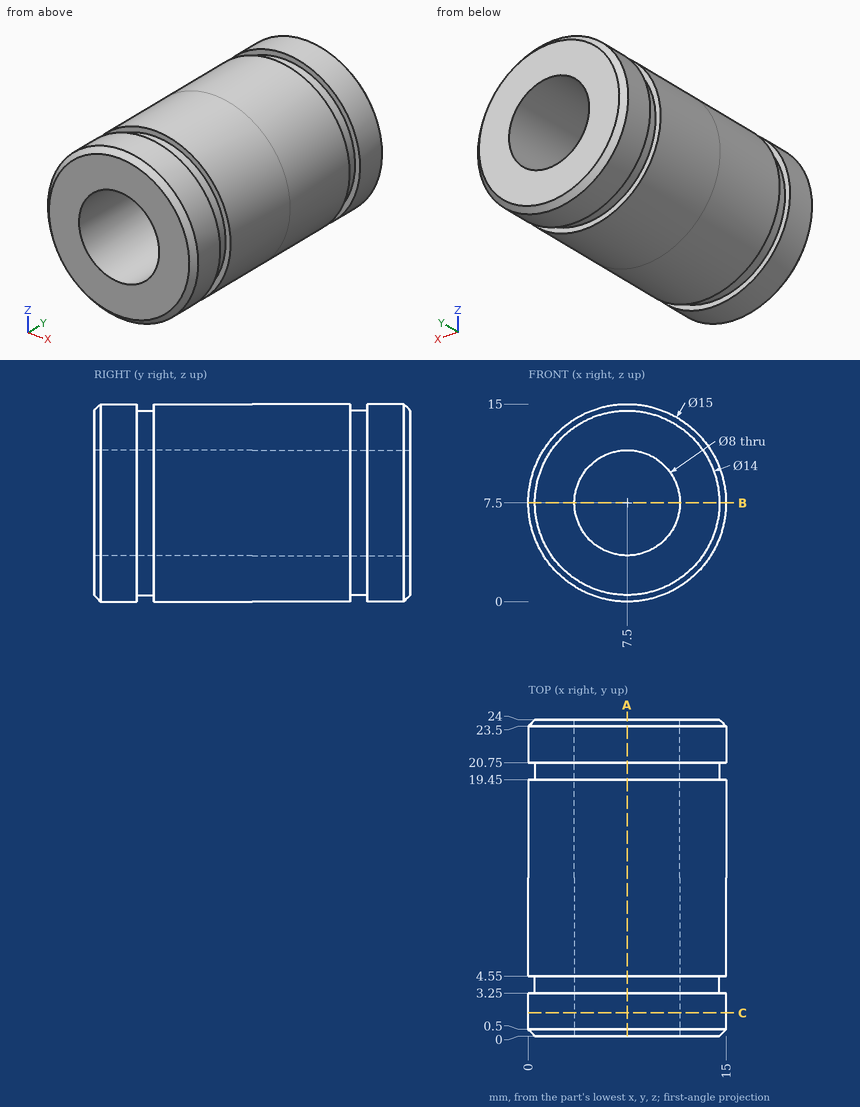
Verification items for this drawing (mm, ordinates from the low corner). Coordinates: 2 decimals unless noted, no trailing zeros. Order: outer loops, then holes, each group sorted by start corner. A loop starts at its lowest first (then second) coordinate and runs counter-clockwise, first axis right, second up. Notation, with made-up numbers: M 51,22 L 107,22 A18 ccw 107,53 Z; hole C 45.5,14 d7. An arc over 180 degrees is marked long. One line per item, written item: value. Start each with the question number.
Item 1: Sectioned sample at B-B on z = 7.5. Record the cut outline in (x, y), then the cut area to 3 significant figures.
Item 2: Sectioned sample at A-A on x = 7.5. Record the cut outline in (y, z).
Item 3: Sectioned sample at C-C on y = 1.75. Record the cut outline in (x, z), then the cut area to 3 significant figures.
Item 4: Thickness scan on probe 1 along X at (y, z) = (18.75, 7.5); probe 2 along Y at (x, z) = (2.25, 2.75); probe 3 along Y at (x, z) = (13.75, 11.25). Record the ranges inside material, lowest first.
Item 5: Depth check by flat-ended pin: P1, Ø1.5, axis at y = 15.5, z = 4.5, coming from the +X side; P2, Ø2, axis at x = 6.5, z = 9.5, coming from the -Y side; P3, Ø5, axis at x = 4, y = 6, coming from the +Z side; P4, Ø3, axis at x = 9.5, z = 5, coming from the +Y side. Enter the tip coordinate at first touch or a pass-through.
Calculated:
1. outline: M 0,0.5 L 0.5,0 L 3.5,0 L 3.5,24 L 0.5,24 L 0,23.5 L 0,20.75 L 0.5,20.75 L 0.5,19.45 L 0,19.45 L 0,4.55 L 0.5,4.55 L 0.5,3.25 L 0,3.25 Z; M 11.5,0 L 14.5,0 L 15,0.5 L 15,3.25 L 14.5,3.25 L 14.5,4.55 L 15,4.55 L 15,19.45 L 14.5,19.45 L 14.5,20.75 L 15,20.75 L 15,23.5 L 14.5,24 L 11.5,24 Z
1. area: 165 mm^2
2. outline: M 0,0.5 L 0.5,0 L 3.25,0 L 3.25,0.5 L 4.55,0.5 L 4.55,0 L 19.45,0 L 19.45,0.5 L 20.75,0.5 L 20.75,0 L 23.5,0 L 24,0.5 L 24,3.5 L 0,3.5 Z; M 0,11.5 L 24,11.5 L 24,14.5 L 23.5,15 L 20.75,15 L 20.75,14.5 L 19.45,14.5 L 19.45,15 L 4.55,15 L 4.55,14.5 L 3.25,14.5 L 3.25,15 L 0.5,15 L 0,14.5 Z
3. outline: C 7.5,7.5 d15; hole C 7.5,7.5 d8
3. area: 126 mm^2
4. probe 1: 0 to 3.5, 11.5 to 15
4. probe 2: 0.08 to 3.25, 4.55 to 19.45, 20.75 to 23.92
4. probe 3: 0.29 to 3.25, 4.55 to 19.45, 20.75 to 23.71
5. P1: x = 14.65
5. P2: through
5. P3: z = 14.93
5. P4: y = 24
